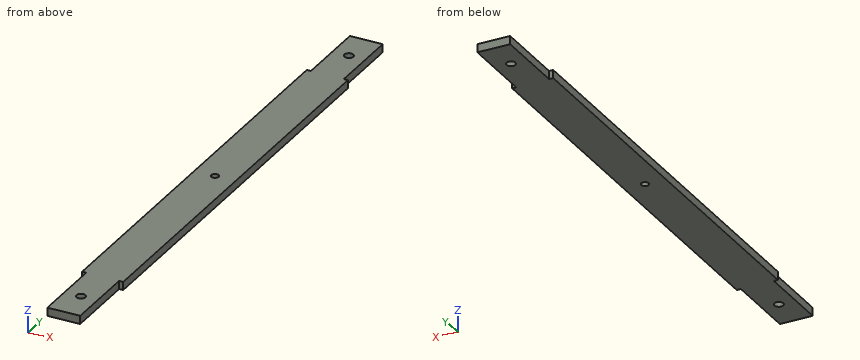
Solid Edge part; units mm, degrees
sketch "Sketch1" plane through (0, 0, 0) normal (0, -1, 0) x (1, 0, 0)
  line L0 (-12.5, -2.5) -> (12.5, -2.5)
  line L1 (12.5, -2.5) -> (12.5, 2.5)
  line L2 (12.5, 2.5) -> (-12.5, 2.5)
  line L3 (-12.5, 2.5) -> (-12.5, -2.5)
  dimension "D1" = 12.5
  dimension "D2" = 12.5
extrude "Protrusion1" add sketch "Sketch1" along normal mid plane 350
sketch "Sketch2" plane through (0, 0, 2.5) normal (0, 0, 1) x (0, 1, 0)
  circle A0 centre (0, 0) radius 2.25
extrude "Cutout1" cut sketch "Sketch2" against normal through all
sketch "Sketch3" plane through (0, 0, -2.5) normal (0, 0, -1) x (0, -1, 0)
  circle A0 centre (-155, 0) radius 2.75
  circle A1 centre (155, 0) radius 2.75
  dimension "D1" = 155
extrude "Cutout2" cut sketch "Sketch3" against normal through all
sketch "Sketch4" plane through (0, 0, -2.5) normal (0, 0, -1) x (0, -1, 0)
  line L0 (-175, 12.5) -> (-130, 12.5)
  line L1 (-130, 12.5) -> (-130, 10)
  line L2 (-130, 10) -> (-175, 10)
  line L3 (-175, 10) -> (-175, 12.5)
  line L4 (-175, -12.5) -> (-130, -12.5)
  line L5 (-130, -12.5) -> (-130, -10)
  line L6 (-130, -10) -> (-175, -10)
  line L7 (-175, -10) -> (-175, -12.5)
  dimension "D1" = 175
extrude "Cutout3" cut sketch "Sketch4" against normal through all
mirror "Mirror1" about plane through (0, 0, 0) normal (0, -1, 0) of "Cutout3"
properties material "AlSi7Mg"
The listing builds one solid part. Answer for the finished solid, in the listing's coordinates (mm). Coordinates: 2 decimals unless noted, no trailing zeros. Write each loop counter-clockwise with the first axis right and the second up, starting at its lowest first coordinate (ties: lowest second). Pieces come first, ordered by that corner, then holes. Notation, with made-up numbers: (-29.5, 18) - (-14.5, 18) arc R22 cw to (-14.5, 54) - close; hole circle Ø7 at (41, 73). An arc over 180 degrees is marked (long way). Return JSON: item names as keys, results as strings. Group by question number.
1. Given pin 1 (2.5 mm diameter, centred on y = -160, z = -0.5, fed in from -X); pin 2 (1.5 mm diameter, centred on y = 144.5, z = 0.5, fed in from +X); pin 3 (0.8 mm diameter, centred on x = -11.5, z = -1, fed in from +Y), each flat-ended and moving along its own axis, determine where each tip first touches the part or whether it passes through.
2. A cutting plane is placed at A-A, the plane z = -1.35. Determine the outline of the cut face in (x, y), plus the area to 3 significant figures.
3. Straight lines are drawn through the part: L1, parallel to Y at x = 0, z = 1.2; L2, parallel to X at y = -155, z = 0.8; L3, parallel to X at y = 0, z = 1. For each, find the intervals that lie inside material, in ascending order.
Ans:
{
 "1": {"pin 1": "x = -10", "pin 2": "x = 10", "pin 3": "y = 130"},
 "2": {"outline": "(-12.5, -130) - (-10, -130) - (-10, -175) - (10, -175) - (10, -130) - (12.5, -130) - (12.5, 130) - (10, 130) - (10, 175) - (-10, 175) - (-10, 130) - (-12.5, 130) - close; hole circle Ø5.5 at (0, -155); hole circle Ø5.5 at (0, 155); hole circle Ø4.5 at (0, 0)", "area": "8,240 mm²"},
 "3": {"L1": "-175 to -157.75, -152.25 to -2.25, 2.25 to 152.25, 157.75 to 175", "L2": "-10 to -2.75, 2.75 to 10", "L3": "-12.5 to -2.25, 2.25 to 12.5"}
}
